Work out the finished part from the listing and answer in its coordinate system (mm). A direction names the side the tool comes from. Round coordinates to 2 decimals unless told otherwise and drop trailing zeros. Write each loop counter-clockwise with the first axis right and the second up, starting at its lowest first coordinate (ties: lowest second). Pieces come first, ordered by that corner, then holes. Notation, with made-up numbers: (56, 20.25) -> (87, 20.25) arc R29 ccw to (87, 45.25) -> close; hole circle Ø10 at (5, 53). An arc over 180 degrees is marked (long way). One line per question, with ' | ' between items. Start each with the question number.
```python
from build123d import *

# Parameters (mm, degrees)
IZIM1_W                     = 60
IZIM1_H                     = 60
Y_KSEKLIK_EKSTR_ZYON1_DEPTH = 70
KES_EKSTR_ZYON1_DEPTH       = 70
IZIM3_W                     = 10
IZIM3_H                     = 30
KES_EKSTR_ZYON2_DEPTH       = 70
IZIM4_W                     = 20
IZIM4_H                     = 30
KES_EKSTR_ZYON5_DEPTH       = 70
IZIM5_W                     = 20
IZIM5_H                     = 15
KES_EKSTR_ZYON6_DEPTH       = 40


with BuildPart() as part:
    # Çizim1 → Yükseklik-Ekstrüzyon1 (new body)
    with BuildSketch(Plane.XY):
        with Locations((-5.635360797, -4.69273743)):
            Rectangle(IZIM1_W, IZIM1_H)
    extrude(amount=Y_KSEKLIK_EKSTR_ZYON1_DEPTH)

    # Çizim2 → Kes-Ekstrüzyon1 (cut)
    with BuildSketch(Plane.XY.offset(70)):
        Polygon((9.364639203, -24.69273743), (1.864639203, -24.69273743), (1.864639203, -34.69273743), (-5.635360797, -34.69273743), (-13.135360797, -34.69273743), (-13.135360797, -24.69273743), (-20.635360797, -24.69273743), (-20.635360797, -14.69273743), (9.364639203, -14.69273743), align=None)
    extrude(amount=-KES_EKSTR_ZYON1_DEPTH, mode=Mode.SUBTRACT)

    # Çizim3 → Kes-Ekstrüzyon2 (cut)
    with BuildSketch(Plane.XY.offset(70)):
        with Locations((19.364639203, 10.30726257)):
            Rectangle(IZIM3_W, IZIM3_H)
        with Locations((-30.635360797, 10.30726257)):
            Rectangle(IZIM3_W, IZIM3_H)
    extrude(amount=-KES_EKSTR_ZYON2_DEPTH, mode=Mode.SUBTRACT)

    # Çizim4 → Kes-Ekstrüzyon5 (cut)
    with BuildSketch(Plane.XY.offset(70)):
        with Locations((-5.635360797, 10.30726257)):
            Rectangle(IZIM4_W, IZIM4_H)
    extrude(amount=-KES_EKSTR_ZYON5_DEPTH, mode=Mode.SUBTRACT)

    # Çizim5 → Kes-Ekstrüzyon6 (cut)
    with BuildSketch(Plane.ZY.offset(25.635360797)):
        with Locations((35, 17.80726257)):
            Rectangle(IZIM5_W, IZIM5_H)
    extrude(amount=-KES_EKSTR_ZYON6_DEPTH, mode=Mode.SUBTRACT)


solid = part.part
```
(1) A cutting plane is placed at B-B, the plane y = 17.5. Determine the outline of the cut face in (x, z), then the cut area to 3 significant figures.
(2) For faces 1 (the flat face through (9, 18, 45)), 2 (the flat face through (-15.635, 10, 35)), 3 (the flat face through (-17, -24.693, 35)), 4 (the flat face through (-25.635, 10, 35)), 5 (the flat face through (19, -4.693, 35)), determine the directions among +Z, -Z, +X, -X, +Y, -Y from which every point of the face is accessible in a straight line to the end or side of a thin tool.
(3) Given pin 1 Ø1.5 at (x, z) = (-10, 60.5) entering from -Y; pin 2 Ø6 at (y, z) = (0, 14.5) entering from +X; pin 3 Ø4 at (x, z) = (-16.5, 33) entering from +Y, each flat-ended and moving along its own axis, determine where each tip first touches the part or whether it passes through.
(4) Consider L1, parallel to X at y = -3, z = 27; L2, parallel to X at y = -21, z = 51.5; L3, parallel to Y at x = 2.5, z = 59. Determine where each line is inside the solid, lowest interval first.
(5) A cutting plane is placed at C-C, the plane z = 21. Determine the outline of the cut face in (x, y), then the cut area to 3 significant figures.
(6) The mould has two halves that part along Y. Classify faces 6 (the flat face through (-31, -4.693, 35)), 7 (the flat face through (6, -24.693, 35)), 8 (the flat face through (13, -34.693, 35)), 9 (the flat face through (-13.135, -30, 35)): +Y half, -Y half, draft (parallel to the pull), parting line (faces both ways), or undercut.
(7) A cutting plane is placed at A-A, the plane y = -22. Determine the outline of the cut face in (x, z), then the cut area to 3 significant figures.
(8) A cutting plane is placed at D-D, the plane x = -29. Determine the outline of the cut face in (y, z), then the cut area to 3 significant figures.
Returned:
1) outline: (-25.64, 0) -> (-15.64, 0) -> (-15.64, 25) -> (-25.64, 25) -> close; (-25.64, 45) -> (-15.64, 45) -> (-15.64, 70) -> (-25.64, 70) -> close; (4.36, 0) -> (14.36, 0) -> (14.36, 25) -> (4.36, 25) -> close; (4.36, 45) -> (14.36, 45) -> (14.36, 70) -> (4.36, 70) -> close | area: 1,000 mm2
2) face 1: +X, -X, +Y | face 2: +Z, -Z, +Y | face 3: +Z, -Z | face 4: +Z, -Z, -X, +Y | face 5: +Z, -Z, +X, +Y
3) pin 1: y = -14.69 | pin 2: x = 14.36 | pin 3: y = 10.31
4) L1: -25.64 to -15.64, 4.36 to 14.36 | L2: -35.64 to -20.64, 9.36 to 24.36 | L3: -34.69 to -24.69, -14.69 to -4.69
5) outline: (-35.64, -34.69) -> (-13.14, -34.69) -> (-13.14, -24.69) -> (-20.64, -24.69) -> (-20.64, -14.69) -> (9.36, -14.69) -> (9.36, -24.69) -> (1.86, -24.69) -> (1.86, -34.69) -> (24.36, -34.69) -> (24.36, -4.69) -> (14.36, -4.69) -> (14.36, 25.31) -> (4.36, 25.31) -> (4.36, -4.69) -> (-15.64, -4.69) -> (-15.64, 25.31) -> (-25.64, 25.31) -> (-25.64, -4.69) -> (-35.64, -4.69) -> close | area: 1,950 mm2
6) face 6: +Y half | face 7: undercut | face 8: -Y half | face 9: draft
7) outline: (-35.64, 0) -> (-20.64, 0) -> (-20.64, 70) -> (-35.64, 70) -> close; (9.36, 0) -> (24.36, 0) -> (24.36, 70) -> (9.36, 70) -> close | area: 2,100 mm2
8) outline: (-34.69, 0) -> (-4.69, 0) -> (-4.69, 70) -> (-34.69, 70) -> close | area: 2,100 mm2
